Here's how the part is built. I have some questions about the finished solid (model axes, mm). Round coordinates to 2 decimals unless told otherwise and drop trailing zeros. Write each loop counter-clockwise with the first axis right and the second up, starting at its lowest first coordinate (ties: lowest second). Pieces come first, ordered by that corner, then holes. Notation, with made-up numbers: (55.25, -26) - (65.25, -26) arc R21 ccw to (65.25, -18) - close; hole circle Ø6 at (81.25, 48). An arc over 180 degrees is marked (long way). Write item = value, one per line. Start each with the question number.
Item 1: If we section it at A-A (x = -4.5): Please give me the cut outline in (y, z), and give its area (3 significant figures).
Item 2: If I drill on line 1 along X through (y, z) = (-4, 74); line 2 along X through (y, z) = (-6.7, 7), over which ranges is the centre line in solid material (lowest first)? Write a range as [from, to].
Item 3: If we section it at C-C (z = 23): Please give me the cut outline in (x, y), and give its area (3 significant figures).
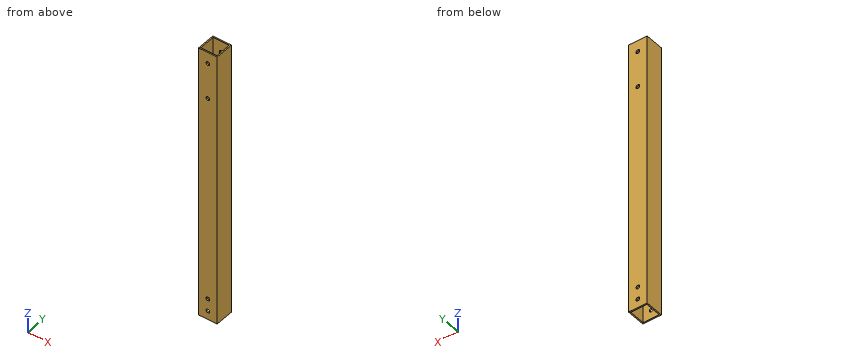
```python
from build123d import *

# Parameters (mm, degrees)
SKETCH1_W           = 15
SKETCH1_H           = 15
SKETCH1_W_2         = 13
SKETCH1_H_2         = 13
BOSS_EXTRUDE1_DEPTH = 221
SKETCH4_R           = 1.5
CUT_EXTRUDE1_DEPTH  = 26
CUT_EXTRUDE2_DEPTH  = 34


with BuildPart() as part:
    # Sketch1 → Boss-Extrude1 (new body)
    with BuildSketch(Plane.XY):
        Rectangle(SKETCH1_W, SKETCH1_H)
        Rectangle(SKETCH1_W_2, SKETCH1_H_2, mode=Mode.SUBTRACT)
    extrude(amount=BOSS_EXTRUDE1_DEPTH)

    # Sketch4 → Cut-Extrude1 (cut)
    with BuildSketch(Plane(origin=(0, 7.5, 0), x_dir=(1, 0, 0), z_dir=(0, 1, 0))):
        with Locations(Location((0, -7, 0), (0, 0, 270))):
            Circle(SKETCH4_R)
        with Locations(Location((0, -17, 0), (0, 0, 270))):
            Circle(SKETCH4_R)
    extrude(amount=-CUT_EXTRUDE1_DEPTH, mode=Mode.SUBTRACT)

    # Sketch5 → Cut-Extrude2 (cut)
    with BuildSketch(Plane(origin=(0, 7.5, 0), x_dir=(1, 0, 0), z_dir=(0, 1, 0))):
        with BuildLine():
            ThreePointArc((1.5, -211.85171377), (1.060660172, -210.791053598), (0, -210.35171377))
            Line((0, -210.35171377), (0, -213.35171377))
            ThreePointArc((0, -213.35171377), (1.060660172, -212.912373942), (1.5, -211.85171377))
        make_face()
        with BuildLine():
            Line((0, -213.35171377), (0, -210.35171377))
            ThreePointArc((0, -210.35171377), (-1.5, -211.85171377), (0, -213.35171377))
        make_face()
        with BuildLine():
            ThreePointArc((1.5, -182.85171377), (1.060660172, -181.791053598), (0, -181.35171377))
            Line((0, -181.35171377), (0, -184.35171377))
            ThreePointArc((0, -184.35171377), (1.060660172, -183.912373942), (1.5, -182.85171377))
        make_face()
        with BuildLine():
            Line((0, -184.35171377), (0, -181.35171377))
            ThreePointArc((0, -181.35171377), (-1.5, -182.85171377), (0, -184.35171377))
        make_face()
    extrude(amount=-CUT_EXTRUDE2_DEPTH, mode=Mode.SUBTRACT)


solid = part.part
```
Reply:
q1.outline = (-7.5, 0) - (-6.5, 0) - (-6.5, 221) - (-7.5, 221) - close; (6.5, 0) - (7.5, 0) - (7.5, 221) - (6.5, 221) - close
q1.area = 442 mm2
q2.line_1 = [-7.5, -6.5], [6.5, 7.5]
q2.line_2 = [-7.5, -1.5], [1.5, 7.5]
q3.outline = (-7.5, -7.5) - (7.5, -7.5) - (7.5, 7.5) - (-7.5, 7.5) - close; hole (-6.5, -6.5) - (6.5, -6.5) - (6.5, 6.5) - (-6.5, 6.5) - close
q3.area = 56.0 mm2
